Verification items for the finished model (mm, model axes). Face numbers are marked on the shaded views. A direction names the side the tool comes from. Round coordinates to 2 decimals unless told otherwise and drop trailing zeros. Write each loop counter-clockwise with the first axis right and the second up, starting at its lowest first coordinate (ties: lowest second). Pieces come first, ordered by that corner, then holes. Notation, with made-up numbers: (52, -28) -> (90, -28) arc R14 ccw to (90, -24) -> close; hole circle Ø6 at (-6.75, -6). An arc over 180 degrees is marked (long way). Use CSV: the item, a comma, the result in double quotes.
```python
from build123d import *

# Parameters (mm, degrees)
BOSS_EXTRUDE1_DEPTH = 20
SKETCH2_R           = 1.5
SKETCH2_R_2         = 2.5
CUT_EXTRUDE1_DEPTH  = 27
SKETCH3_R           = 1.5
CUT_EXTRUDE2_DEPTH  = 27


with BuildPart() as part:
    # Sketch1 → Boss-Extrude1 (new body)
    with BuildSketch(Plane.XY):
        with BuildLine():
            Line((-1.016707819, -10.4), (20.983292181, -10.4))
            Line((20.983292181, -10.4), (20.983292181, -19.4))
            Line((20.983292181, -19.4), (17.983292181, -19.4))
            Line((17.983292181, -19.4), (17.983292181, -13.4))
            Line((17.983292181, -13.4), (-1.016707819, -13.4))
            ThreePointArc((-1.016707819, -13.4), (-3.491581553, -12.374873734), (-4.516707819, -9.9))
            Line((-4.516707819, -9.9), (-4.516707819, 9.9))
            ThreePointArc((-4.516707819, 9.9), (-3.491581553, 12.374873734), (-1.016707819, 13.4))
            Line((-1.016707819, 13.4), (17.983292181, 13.4))
            Line((17.983292181, 13.4), (17.983292181, 19.4))
            Line((17.983292181, 19.4), (20.983292181, 19.4))
            Line((20.983292181, 19.4), (20.983292181, 10.4))
            Line((20.983292181, 10.4), (-1.016707819, 10.4))
            ThreePointArc((-1.016707819, 10.4), (-1.370261209, 10.253553391), (-1.516707819, 9.9))
            Line((-1.516707819, 9.9), (-1.516707819, -9.9))
            ThreePointArc((-1.516707819, -9.9), (-1.370261209, -10.253553391), (-1.016707819, -10.4))
        make_face()
    extrude(amount=BOSS_EXTRUDE1_DEPTH)

    # Sketch2 → Cut-Extrude1 (cut)
    with BuildSketch(Plane(origin=(0, 13.4, 0), x_dir=(1, 0, 0), z_dir=(0, 1, 0))):
        with Locations((0.983292181, -14)):
            Circle(SKETCH2_R)
        with Locations((9.733292181, -5)):
            Circle(SKETCH2_R_2)
    extrude(amount=-CUT_EXTRUDE1_DEPTH, mode=Mode.SUBTRACT)

    # Sketch3 → Cut-Extrude2 (cut)
    with BuildSketch(Plane.ZY.offset(-17.983292181)):
        with Locations((16, 16.4)):
            Circle(SKETCH3_R)
        with Locations((4, 16.4)):
            Circle(SKETCH3_R)
        with Locations((4, -16.4)):
            Circle(SKETCH3_R)
        with Locations((16, -16.4)):
            Circle(SKETCH3_R)
    extrude(amount=-CUT_EXTRUDE2_DEPTH, mode=Mode.SUBTRACT)


solid = part.part
```
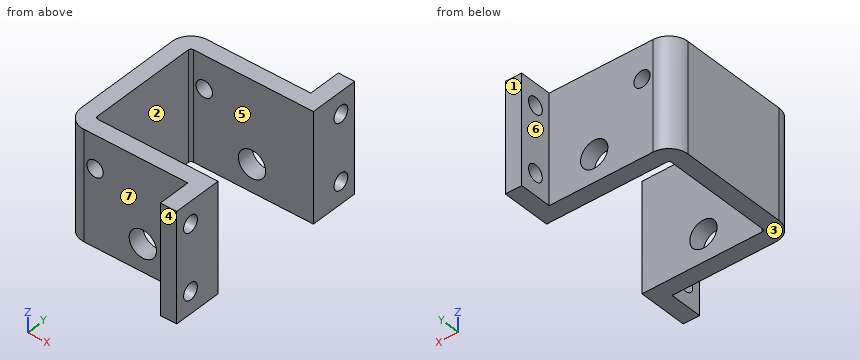
Q1. Go/stop test with flat-tipped pins: P1, Ø6.5, axis at x = 9.73, z = 5, coming from the +Y side; P2, Ø6.5, axis at y = 17, z = 10.5, coming from the -X side; P3, Ø10, axis at y = -3.5, z = 2, coming from the +X side. Record where each tip stops, or that it passes through.
Filled in:
P1,"y = 13.4"
P2,"x = 17.98"
P3,"x = -1.52"
Q2. Access from +Z, -Z, +X, -X, +Y, -Y to the whole of each face (thin tool, end or side, straight path). Record for the marked faces 4, 5, 6 and 7.
Filled in:
face 4,"+Z, -Z, +X, -X, -Y"
face 5,"+Z, -Z, +X"
face 6,"+Z, -Z, -X, +Y"
face 7,"+Z, -Z, -X, -Y"
Q3. Section check A-A (z = 16). Record the cut outline in (x, y).
Filled in:
outline,"(-4.52, -9.9) arc R3.5 ccw to (-1.02, -13.4) -> (17.98, -13.4) -> (17.98, -14.9) -> (20.98, -14.9) -> (20.98, -10.4) -> (-1.02, -10.4) arc R0.5 cw to (-1.52, -9.9) -> (-1.52, 9.9) arc R0.5 cw to (-1.02, 10.4) -> (20.98, 10.4) -> (20.98, 14.9) -> (17.98, 14.9) -> (17.98, 13.4) -> (-1.02, 13.4) arc R3.5 ccw to (-4.52, 9.9) -> close; (17.98, -19.4) -> (20.98, -19.4) -> (20.98, -17.9) -> (17.98, -17.9) -> close; (17.98, 17.9) -> (20.98, 17.9) -> (20.98, 19.4) -> (17.98, 19.4) -> close"
Q4. Section check B-B (y = 15.5). Record the cut outline in (x, z).
Filled in:
outline,"(17.98, 0) -> (20.98, 0) -> (20.98, 2.8) -> (17.98, 2.8) -> close; (17.98, 5.2) -> (20.98, 5.2) -> (20.98, 14.8) -> (17.98, 14.8) -> close; (17.98, 17.2) -> (20.98, 17.2) -> (20.98, 20) -> (17.98, 20) -> close"
Q5. Mould release check, pull along Y, two halves, no side actions. Record for the marked faces 1, 2 and 3: released by +Y, released by -Y, zero draft, split by the parting line, or undercut.
Filled in:
face 1,"released by +Y"
face 2,"undercut"
face 3,"zero draft"
Q6. Material ranges on L1, parallel to Y at x = 19.85, z = 4; L2, parallel to Y at x = -0.75, z = 3; L3, parallel to Y at x = 19.75, z = 12.5, recorded low to high.
Filled in:
L1,"-19.4 to -17.9, -14.9 to -10.4, 10.4 to 14.9, 17.9 to 19.4"
L2,"-13.4 to -10.4, 10.4 to 13.4"
L3,"-19.4 to -10.4, 10.4 to 19.4"
Q7. Section check C-C (x = 3.75). Record the cut outline in (y, z).
Filled in:
outline,"(-13.4, 0) -> (-10.4, 0) -> (-10.4, 20) -> (-13.4, 20) -> close; (10.4, 0) -> (13.4, 0) -> (13.4, 20) -> (10.4, 20) -> close"
Q8. Section check D-D (x = 0.75). Record the cut outline in (y, z).
Filled in:
outline,"(-13.4, 0) -> (-10.4, 0) -> (-10.4, 12.52) -> (-13.4, 12.52) -> close; (-13.4, 15.48) -> (-10.4, 15.48) -> (-10.4, 20) -> (-13.4, 20) -> close; (10.4, 0) -> (13.4, 0) -> (13.4, 12.52) -> (10.4, 12.52) -> close; (10.4, 15.48) -> (13.4, 15.48) -> (13.4, 20) -> (10.4, 20) -> close"
